The figure shows three views and two pictorial views of one solid part (mm, origin at its lowest corner). Answer the questions. Round coordinates to 2 decimals unless told otherwise and drop trailing zeros. Write each loop counter-clockwise with the first axis right and the second up, starting at its lowest first coordinate (ties: lowest second). Pieces come first, ordered by that corner, then holes.
Item 1: Each of these flat-tipped pins is pushed along its axis until it touches: pin 1 (2 mm diameter, centred on x = 6, y = 16.5, fed in from +Z); pin 2 (1.2 mm diameter, centred on x = 16, y = 16, fed in from -Z); pin 3 (2.5 mm diameter, centred on x = 4, y = 4, fed in from +Z). Where does it stop, or does it pass through?
Item 2: Find section C-C on y = 8.5. Give the number of separate pieces and of enclosed holes in the cut face, then the cut area to 3 significant figures.
Item 3: Find section B-B on z = 38.1. Give the vertices of the cut face in (x, y).
Item 4: Find the intervals of material crossed by probe 1 along Y at (x, z) = (4, 23.5); probe 2 along X at (y, z) = (7.25, 127); probe 3 along X at (y, z) = (14.25, 101), in increasing order.
Item 5: Find section A-A on z = 101.6. Give the vertices of the cut face in (x, y).
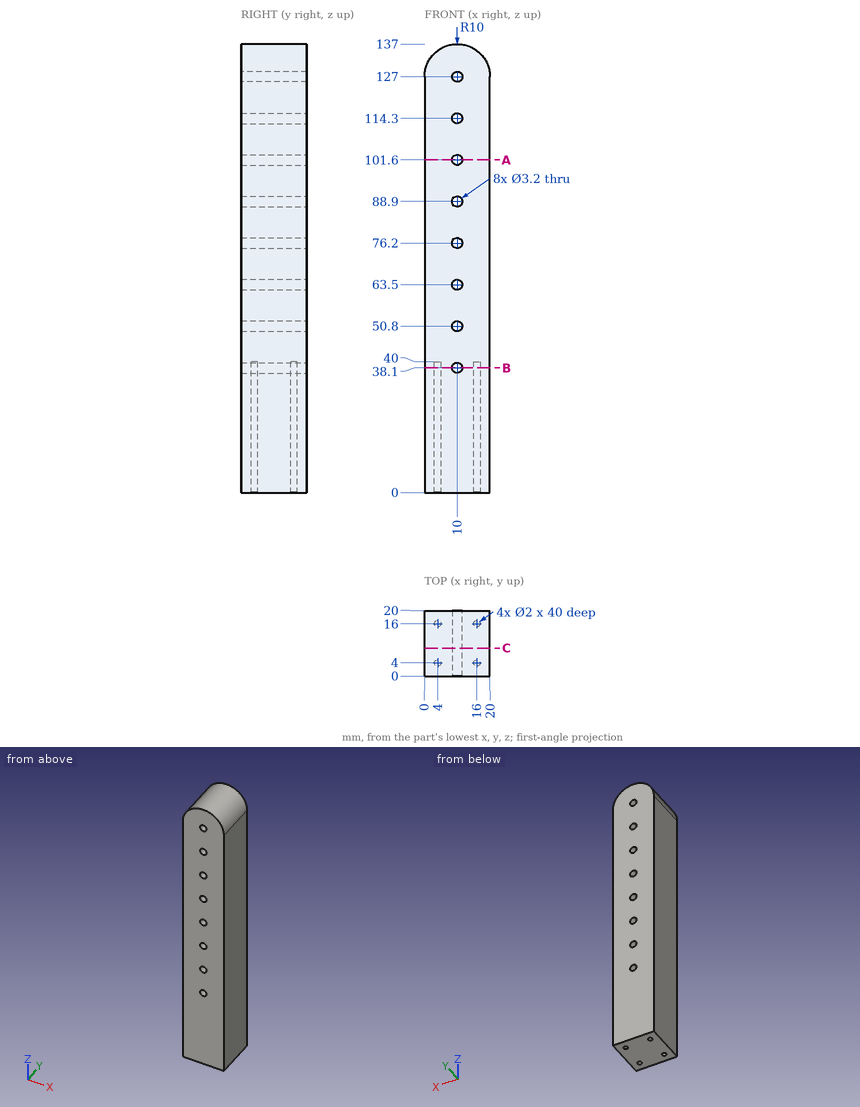
Check values:
1. pin 1: stops at z = 136.54
1. pin 2: stops at z = 40
1. pin 3: stops at z = 135.8
2. separate pieces: 1
2. enclosed holes: 8
2. area: 2,630 mm2
3. outline: (0, 0) - (8.4, 0) - (8.4, 20) - (0, 20) - close; (11.6, 0) - (20, 0) - (20, 20) - (11.6, 20) - close; hole circle Ø2 at (4, 4); hole circle Ø2 at (4, 16); hole circle Ø2 at (16, 4); hole circle Ø2 at (16, 16)
4. probe 1: y = 0 to 3, 5 to 15, 17 to 20
4. probe 2: x = 0 to 8.4, 11.6 to 20
4. probe 3: x = 0 to 8.52, 11.48 to 20
5. outline: (0, 0) - (8.4, 0) - (8.4, 20) - (0, 20) - close; (11.6, 0) - (20, 0) - (20, 20) - (11.6, 20) - close
